from build123d import *

# Parameters (mm, degrees)
SKETCH038_W     = 20
SKETCH038_H     = 28.8
PAD013_DEPTH    = 8
SKETCH039_W     = 9
SKETCH039_H     = 4.5
POCKET025_DEPTH = 28.8
SKETCH040_R     = 1.5
POCKET023_DEPTH = 4
SKETCH041_W     = 20
SKETCH041_H     = 4.95
POCKET026_DEPTH = 0.1


with BuildPart() as part:
    # Sketch038 → Pad013 (new body)
    with BuildSketch(Plane.XY):
        with Locations((-4.5, 14.4)):
            Rectangle(SKETCH038_W, SKETCH038_H)
    extrude(amount=PAD013_DEPTH)

    # Sketch039 (on Face1 of Pad013) → Pocket025 (cut)
    with BuildSketch(Plane.XZ):
        with Locations((-4.5, 2.25)):
            Rectangle(SKETCH039_W, SKETCH039_H)
    extrude(amount=-POCKET025_DEPTH, mode=Mode.SUBTRACT)

    # Sketch040 (on Face8 of Pocket025) → Pocket023 (cut)
    with BuildSketch(Plane.XY.offset(8)):
        with Locations((-12, 19.4)):
            Circle(SKETCH040_R)
        with Locations((3, 9.4)):
            Circle(SKETCH040_R)
        with Locations((-12, 9.4)):
            Circle(SKETCH040_R)
        with Locations((3, 19.4)):
            Circle(SKETCH040_R)
    extrude(amount=-POCKET023_DEPTH, mode=Mode.SUBTRACT)

    # Sketch041 (on Face8 of Pocket023) → Pocket026 (cut)
    with BuildSketch(Plane.XY.offset(8)):
        with Locations((-4.5, 26.325)):
            Rectangle(SKETCH041_W, SKETCH041_H)
        with Locations((-4.5, 2.475)):
            Rectangle(SKETCH041_W, SKETCH041_H)
    extrude(amount=-POCKET026_DEPTH, mode=Mode.SUBTRACT)


with BuildPart() as part_1:
    # Body014 placement: moved
    add(part.part.moved(Location((0, 100, 2))))


solid = part_1.part
Geometry: final body of the model. Coordinates: model frame, mm. A direction names the side the tool comes from. Give positions to 0.01 mm unless a question says otherwise; leave off trailing zeros. Loops run counter-clockwise (first coordinate to the right, second up) from the corner with the lowest first, then second, coordinate; pieces in that order, holes last. Notation, with made-up numbers: M 58.5,69.5 L 83.5,69.5 A23 cw 83.5,86.5 Z; hole C -6.75,63 d4. An arc over 180 degrees is marked long. Put each result on its own line as item: value.
1) First-contact query: P1, Ø2.5, axis at x = -11.5, y = 119.5, coming from the +Z side; P2, Ø1.5, axis at x = -11.5, y = 109, coming from the +Z side; P3, Ø2.5, axis at x = -5.5, y = 103, coming from the +Z side. Flat tips, straight axial feed; report the tip coordinate or a pass-through.
Computed values:
P1: stops at z = 10
P2: stops at z = 6
P3: stops at z = 9.9
2) Reachability of faces 5 (the flat face through (-5, 114, 6.5)), 6 (the flat face through (3, 109, 6)), 7 (the flat face through (-5, 115, 10)), 8 (the flat face through (3, 115, 2)), 9 (the flat face through (-5, 126, 9.9)) from +Z, -Z, +X, -X, +Y, -Y: full face, straight path, thin tool, end or side. Return the list, or none.
Computed values:
face 5: -Z, +Y, -Y
face 6: +Z
face 7: +Z, +X, -X, +Y, -Y
face 8: -Z, +X, -X, +Y, -Y
face 9: +Z, +X, -X, +Y
3) Cut plane B-B, the plane y = 109.4. Return the cut outline in (x, z), plus the area to 3 significant figures.
Computed values:
outline: M -14.5,2 L -9,2 L -9,6.5 L 0,6.5 L 0,2 L 5.5,2 L 5.5,10 L 4.5,10 L 4.5,6 L 1.5,6 L 1.5,10 L -10.5,10 L -10.5,6 L -13.5,6 L -13.5,10 L -14.5,10 Z
area: 95.5 mm^2
4) Cut plane D-D, the plane y = 113. Return the cut outline in (x, z).
Computed values:
outline: M -14.5,2 L -9,2 L -9,6.5 L 0,6.5 L 0,2 L 5.5,2 L 5.5,10 L -14.5,10 Z
5) Material intervals for L1, parallel to Y at x = -12, z = 7.1; L2, parallel to X at y = 119.4, z = 7.8; L3, parallel to X at y = 115, z = 4.5, sorted ascending. Write a range as from..to.
Computed values:
L1: y = 100..107.9, 110.9..117.9, 120.9..128.8
L2: x = -14.5..-13.5, -10.5..1.5, 4.5..5.5
L3: x = -14.5..-9, 0..5.5
6) Mould query, pull axis Y, two halves, no side actions, for faces 1 (the flat face through (3, 119, 6)), 2 (the flat face through (-5, 128.8, 7)), 3 (the flat face through (-12, 109, 6)), 4 (the flat face through (-9, 114, 4)). Classes: released by +Y, released by -Y, zero draft, split by the parting line, or undercut.
Computed values:
face 1: undercut
face 2: released by +Y
face 3: undercut
face 4: zero draft
7) Cut plane A-A, the plane z = 7.5. Return the cut outline in (x, y), plus the area to 3 significant figures.
Computed values:
outline: M -14.5,100 L 5.5,100 L 5.5,128.8 L -14.5,128.8 Z; hole C -12,109.4 d3; hole C -12,119.4 d3; hole C 3,109.4 d3; hole C 3,119.4 d3
area: 548 mm^2
8) Cut plane C-C, the plane x = -12. Return the cut outline in (y, z), plus the area to 3 significant figures.
Computed values:
outline: M 100,2 L 128.8,2 L 128.8,9.9 L 123.85,9.9 L 123.85,10 L 120.9,10 L 120.9,6 L 117.9,6 L 117.9,10 L 110.9,10 L 110.9,6 L 107.9,6 L 107.9,10 L 104.95,10 L 104.95,9.9 L 100,9.9 Z
area: 205 mm^2
